Read the model definition and answer for the solid it produces. Units are mm, in the model's axes. A direction names the side the tool comes from. Coordinates: 2 decimals unless noted, no trailing zeros. Loops run counter-clockwise (first coordinate to the right, second up) from the corner with the lowest first, then second, coordinate; pieces in that order, holes last. Notation, with made-up numbers: (15.25, 0) -> (49.25, 0) arc R20 cw to (49.25, 39) -> close; hole circle Ø4 at (58.5, 21). An arc over 180 degrees is marked (long way). Answer as a JSON object with one key per item and string values. Group by question number.
Q1. Straight lines are drawn through the part: line 1 along Z through (x, y) = (64.5, -18.75) (3 decimals); line 2 along X through (y, z) = (-20.25, 62) (3 decimals); line 3 along X through (y, z) = (-10, -5) (3 decimals). For each, find the intervals that lie inside material, in ascending order. Write a range as [from, to].
Q2. Each of these flat-tipped pins is pushed along its axis until it touches: P1, Ø5, axis at y = -17.5, z = 65, coming from the -X side (3 decimals); P2, Ø10, axis at x = 54, y = -16, coming from the -Z side; P3, Ø8, axis at y = -14, z = 9, coming from the +X side (3 decimals). Where does it stop, or does it pass through?
Q3. The part is cut by section B-B on x = 84. Write down the section's boundary in (y, z) (3 decimals).
Q4. The part is cut by section A-A on z = 0.5. Write down the section's boundary in (x, y) (3 decimals).
Q5. For faces 1 (the flat face through (59, -13, 42.875)), 2 (the flat face through (41.275, -13, 8)), 3 (the flat face through (60.325, -13, 64)), determine the directions among +Z, -Z, +X, -X, +Y, -Y from which every point of the face is accessible in a straight line to the end or side of a thin tool.
from build123d import *

# Parameters (mm, degrees)
F0_W     = 25.4
F0_H     = 4.7498
F0_H_2   = 4.7752
F0_H_3   = 19.05
F1_DEPTH = 25.4


with BuildPart() as f1:
    # F0 (on Front) → F1 (new body)
    with BuildSketch(Plane.XZ):
        Polygon((-41.275, 9.525), (-41.275, -9.525), (41.275, -9.525), (41.275, 9.525), (22.225, 9.525), align=None)
        with BuildLine():
            add(Edge.make_bspline(
                [(-41.275, 9.525), (-41.9137682091, 44.8755109518), (19.7088872763, 61.1237978396), (55.9633224652, 61.9050337831)],
                knots=[0, 0, 0, 0, 110.2917325218, 110.2917325218, 110.2917325218, 110.2917325218], degree=3))
            Line((-41.275, 9.525), (22.225, 9.525))
            Line((22.225, 9.525), (22.225, 27.0002))
            ThreePointArc((22.225, 27.0002), (32.0382463983, 51.2727247152), (55.9633224652, 61.9050337831))
        make_face()
        with Locations((73.025, 64.3001)):
            Rectangle(F0_W, F0_H)
        with Locations((73.025, 40.4876)):
            Rectangle(F0_W, F0_H_2)
        Polygon((85.725, 66.675), (85.725, 61.9252), (85.725, 42.8752), (85.725, 38.1), (111.125, 38.1), (111.125, 66.675), align=None)
        with BuildLine():
            Line((22.225, 9.525), (41.275, 9.525))
            Line((41.275, 9.525), (41.275, 27.0002))
            ThreePointArc((41.275, 27.0002), (45.9246798487, 38.2255201513), (57.15, 42.8752))
            Line((57.15, 42.8752), (60.325, 42.8752))
            Line((60.325, 42.8752), (60.325, 61.9252))
            Line((60.325, 61.9252), (57.15, 61.9252))
            add(Edge.make_bspline(
                [(55.9633224652, 61.9050337831), (56.3619879863, 61.9136245068), (56.757586004, 61.9203449679), (57.15, 61.9252)],
                knots=[110.2917325218, 110.2917325218, 110.2917325218, 110.2917325218, 111.5045361635, 111.5045361635, 111.5045361635, 111.5045361635], degree=3))
            ThreePointArc((55.9633224652, 61.9050337831), (32.0382463983, 51.2727247152), (22.225, 27.0002))
            Line((22.225, 27.0002), (22.225, 9.525))
        make_face()
        with Locations((73.025, 52.4002)):
            Rectangle(F0_W, F0_H_3)
    extrude(amount=F1_DEPTH)


solid = f1.part
Final values:
{
 "1": {"line 1": "z = [38.1, 66.675]", "line 2": "x = [60.325, 111.125]", "line 3": "x = [-41.275, 41.275]"},
 "2": {"P1": "stops at x = 60.325", "P2": "stops at z = 40.62", "P3": "stops at x = 41.275"},
 "3": {"outline": "(-25.4, 38.1) -> (0, 38.1) -> (0, 66.675) -> (-25.4, 66.675) -> close"},
 "4": {"outline": "(-41.275, -25.4) -> (41.275, -25.4) -> (41.275, 0) -> (-41.275, 0) -> close"},
 "5": {"face 1": "-Z, +Y, -Y", "face 2": "-Z, +X, +Y, -Y", "face 3": "+Z, -X, +Y, -Y"}
}
